Check sheet for the modelled part. Datum: model origin and axes. Units: mm. Coordinates: 2 decimals unless noted, no trailing zeros. Order: outer loops, then holes, each group sorted by start corner. A loop starts at its lowest first (then second) coordinate and runs counter-clockwise, first axis right, second up.
1. Gauge pin test, flat ends, axial feed: pin 1 Ø1.5 at (y, z) = (4, 3) entering from -X; pin 2 Ø2.5 at (y, z) = (16, 3.5) entering from +X; pin 3 Ø1.5 at (y, z) = (31, 2.5) entering from -X. Record the tip position at first contact, or that the pin passes through.
2. Cross-section at C-C (x = 42.5). Enter the section's corners in (y, z), then the cut area to 3 significant figures.
3. Thickness scan on line 1 (Y direction, x = 0, z = 1.5); line 2 (X direction, y = 3, z = 3.1); line 3 (X direction, y = -8, z = 3.25). Record the ranges inside material, lowest first.
4. Cross-section at B-B (z = 2.1). Enter the section's corners in (x, y).
5. Cross-section at A-A (y = 0). Enter the section's corners in (x, z).
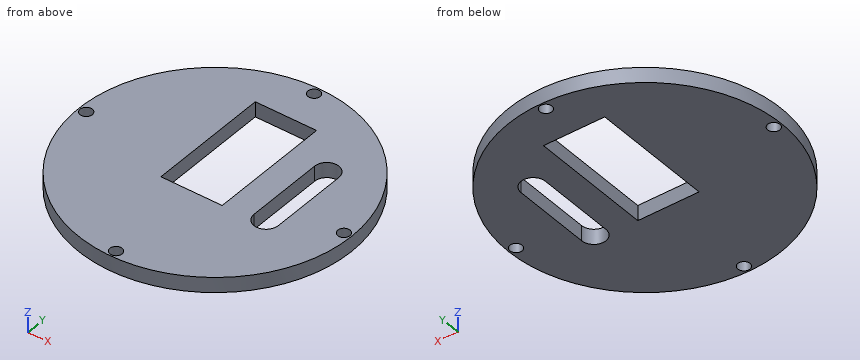
```python
from build123d import *

# Parameters (mm, degrees)
SKETCH1_R           = 45
SKETCH1_R_2         = 2
SKETCH1_W           = 20.2
SKETCH1_H           = 40.5
BOSS_EXTRUDE1_DEPTH = 5
CUT_EXTRUDE1_DEPTH  = 10


with BuildPart() as part:
    # Sketch1 → Boss-Extrude1 (new body)
    with BuildSketch(Plane.XY):
        Circle(SKETCH1_R)
        with Locations((42.5, 0)):
            Circle(SKETCH1_R_2, mode=Mode.SUBTRACT)
        with Locations((0, -42.5)):
            Circle(SKETCH1_R_2, mode=Mode.SUBTRACT)
        with Locations((-42.5, 0)):
            Circle(SKETCH1_R_2, mode=Mode.SUBTRACT)
        with Locations((0, 42.5)):
            Circle(SKETCH1_R_2, mode=Mode.SUBTRACT)
        with Locations((0, 10.15)):
            Rectangle(SKETCH1_W, SKETCH1_H, mode=Mode.SUBTRACT)
    extrude(amount=BOSS_EXTRUDE1_DEPTH)

    # Sketch2 → Cut-Extrude1 (cut)
    with BuildSketch(Plane(origin=(0, 0, 0), x_dir=(-1, 0, 0), z_dir=(0, 0, -1))):
        with BuildLine():
            Line((-19, 18), (-19, -8))
            ThreePointArc((-19, -8), (-23, -12), (-27, -8))
            Line((-27, -8), (-27, 18))
            ThreePointArc((-27, 18), (-23, 22), (-19, 18))
        make_face()
    extrude(amount=-CUT_EXTRUDE1_DEPTH, mode=Mode.SUBTRACT)


solid = part.part
```
Data:
1. pin 1: stops at x = -44.88
1. pin 2: stops at x = 42.51
1. pin 3: stops at x = -33.32
2. outline: (-14.79, 0) - (-2, 0) - (-2, 5) - (-14.79, 5) - close; (2, 0) - (14.79, 0) - (14.79, 5) - (2, 5) - close
2. area: 128 mm2
3. line 1: y = -45 to -44.5, -40.5 to -10.1, 30.4 to 40.5, 44.5 to 45
3. line 2: x = -44.9 to -10.1, 10.1 to 19, 27 to 44.9
3. line 3: x = -44.28 to -10.1, 10.1 to 19, 27 to 44.28
4. outline: circle Ø90 at (0, 0); hole circle Ø4 at (-42.5, 0); hole (-10.1, -10.1) - (10.1, -10.1) - (10.1, 30.4) - (-10.1, 30.4) - close; hole circle Ø4 at (0, -42.5); hole circle Ø4 at (0, 42.5); hole (19, -8) arc R4 ccw to (27, -8) - (27, 18) arc R4 ccw to (19, 18) - close; hole circle Ø4 at (42.5, 0)
5. outline: (-45, 0) - (-44.5, 0) - (-44.5, 5) - (-45, 5) - close; (-40.5, 0) - (-10.1, 0) - (-10.1, 5) - (-40.5, 5) - close; (10.1, 0) - (19, 0) - (19, 5) - (10.1, 5) - close; (27, 0) - (40.5, 0) - (40.5, 5) - (27, 5) - close; (44.5, 0) - (45, 0) - (45, 5) - (44.5, 5) - close
